Work out the finished part from the listing and answer in its coordinate system (mm). Round coordinates to 2 decimals unless told otherwise and drop trailing zeros. Write each loop counter-clockwise with the first axis right and the second up, starting at its lowest first coordinate (ties: lowest second). Pieces come first, ordered by that corner, then holes. Notation, with made-up numbers: (35.25, 34) -> (63.25, 34) arc R10 ccw to (63.25, 40) -> close; hole circle Ø1 at (38.5, -24). An arc over 180 degrees is marked (long way). One line per item, written item: value.
```python
from build123d import *

# Parameters (mm, degrees)
F0_W     = 40
F0_H     = 40
F1_DEPTH = 200
F2_W     = 20
F2_H     = 15
F3_DEPTH = 40.001
F4_W     = 20
F4_H     = 15
F5_DEPTH = 40.001
F6_W     = 20
F6_H     = 20
F7_DEPTH = 195.001


with BuildPart() as f1:
    # F0 (on Top) → F1 (new body)
    with BuildSketch(Plane.XY):
        Rectangle(F0_W, F0_H)
    extrude(amount=F1_DEPTH)

    # F2 (on face) → F3 (cut, through all)
    with BuildSketch(Plane.YZ.offset(20)):
        with Locations((0, 12.5)):
            Rectangle(F2_W, F2_H)
        with Locations((0, 32.5)):
            Rectangle(F2_W, F2_H)
        with Locations((0, 52.5)):
            Rectangle(F2_W, F2_H)
        with Locations((0, 72.5)):
            Rectangle(F2_W, F2_H)
        with Locations((0, 92.5)):
            Rectangle(F2_W, F2_H)
        with Locations((0, 112.5)):
            Rectangle(F2_W, F2_H)
        with Locations((0, 132.5)):
            Rectangle(F2_W, F2_H)
        with Locations((0, 152.5)):
            Rectangle(F2_W, F2_H)
        with Locations((0, 172.5)):
            Rectangle(F2_W, F2_H)
        with Locations((0, 192.5)):
            Rectangle(F2_W, F2_H)
    extrude(amount=-F3_DEPTH, mode=Mode.SUBTRACT)

    # F4 (on face) → F5 (cut, through all)
    with BuildSketch(Plane.XZ.offset(20)):
        with Locations((0, 12.5)):
            Rectangle(F4_W, F4_H)
        with Locations((0, 32.5)):
            Rectangle(F4_W, F4_H)
        with Locations((0, 52.5)):
            Rectangle(F4_W, F4_H)
        with Locations((0, 72.5)):
            Rectangle(F4_W, F4_H)
        with Locations((0, 92.5)):
            Rectangle(F4_W, F4_H)
        with Locations((0, 112.5)):
            Rectangle(F4_W, F4_H)
        with Locations((0, 132.5)):
            Rectangle(F4_W, F4_H)
        with Locations((0, 152.5)):
            Rectangle(F4_W, F4_H)
        with Locations((0, 172.5)):
            Rectangle(F4_W, F4_H)
        with Locations((0, 192.5)):
            Rectangle(F4_W, F4_H)
    extrude(amount=-F5_DEPTH, mode=Mode.SUBTRACT)

    # F6 (on face) → F7 (cut, through all)
    with BuildSketch(Plane.XY.offset(5)):
        Rectangle(F6_W, F6_H)
    extrude(amount=F7_DEPTH, mode=Mode.SUBTRACT)


solid = f1.part
```
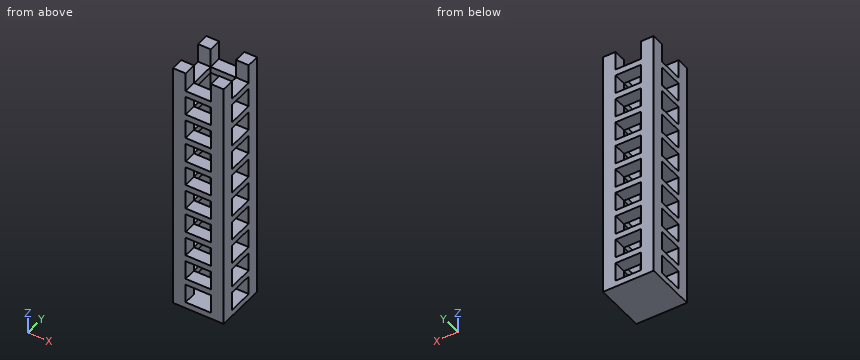
(1) Find section A-A on z = 188. Give the vertices of the cut face in (x, y), plus the area to 3 significant figures.
Reported:
outline: (-20, -20) -> (-10, -20) -> (-10, -10) -> (-20, -10) -> close; (-20, 10) -> (-10, 10) -> (-10, 20) -> (-20, 20) -> close; (10, -20) -> (20, -20) -> (20, -10) -> (10, -10) -> close; (10, 10) -> (20, 10) -> (20, 20) -> (10, 20) -> close
area: 400 mm2
(2) Find section C-C on y = -7. Give the number of separate pieces and of enclosed holes in the cut face, plus the area to 3 significant figures.
Reported:
separate pieces: 19
enclosed holes: 0
area: 1,100 mm2
(3) Find section B-B on z = 83. Give the vertices of the cut face in (x, y), plus the area to 3 significant figures.
Reported:
outline: (-20, -20) -> (20, -20) -> (20, 20) -> (-20, 20) -> close; hole (-10, -10) -> (10, -10) -> (10, 10) -> (-10, 10) -> close
area: 1,200 mm2
(4) Consider probe 1 along X at (y, z) = (16.5, 130.5); probe 2 along Z at (x, y) = (-0.5, -9.5). Determine where each line is inside the solid, lowest interval first.
Reported:
probe 1: x = -20 to -10, 10 to 20
probe 2: z = 0 to 5
(5) A flat-ended cylindrical pin translates along its axis: pin 1 Ø5 at (x, y) = (-17.5, 1.5) entering from +Z. Find the tip coordinate at first contact, or state that the pin passes through.
Reported:
pin 1: stops at z = 185
